from build123d import *


with BuildPart() as part:
    # Sketch1 one side → Revolve1 (revolve)
    with BuildSketch(Plane.XY, mode=Mode.PRIVATE) as revolve1_sk:
        Polygon((0, -3.175), (0, 6.35), (-3.175, 6.35), (-3.175, 5.715), (-2.8575, 5.715), (-2.8575, -2.921), (-2.6035, -3.175), align=None)
    revolve(revolve1_sk.sketch.rotate(Axis((0, 0, 0), (0, 1, 0)), 180), axis=Axis((0, 0, 0), (0, 1, 0)))  # turned: the seam where the file's is

    # Sketch2 → #6-80 Tapped Hole1 (revolve, cut)
    with BuildSketch(Plane(origin=(0, 6.35, 0), x_dir=(0, 0, 1), z_dir=(1, 0, 0))):
        Polygon((0, 0), (0, 9.525), (1.5748, 9.525), (1.3208, 8.911789755), (1.3208, 0.613210245), (1.5748, 0), align=None)
    revolve(axis=Axis((0, 12.7, 0), (0, -1, 0)), mode=Mode.SUBTRACT)


solid = part.part
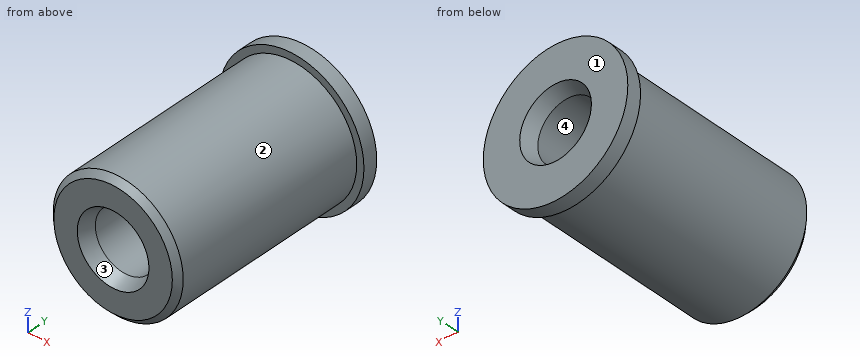
Verification items for the finished model (mm, model axes). Face numbers are marked on the shaded views. Round coordinates to 2 decimals unless told otherwise and drop trailing zeros. Loops run counter-clockwise (first coordinate to the right, second up) from the corner with the lowest first, then second, coordinate; pieces in that order, holes last. Notation, with made-up numbers: (71.25, -8.5) - (84.25, -8.5) arc R21 ccw to (84.25, 23.5) - close; hole circle Ø5 at (-36.75, 10). An arc over 180 degrees is marked (long way). Write item = value, one per line.
Q1. Depth check by flat-ended pin: pin 1 (3 mm diameter, centred on x = -2, y = -2, fed in from -Z); pin 2 (1.5 mm diameter, centred on x = 0.5, y = 2.5, fed in from +Z); pin 3 (2 mm diameter, centred on y = 1.5, z = -0.5, fed in from +X). Enter the tip coordinate at first touch or a pass-through.
Here are the results:
pin_1 = -2.81
pin_2 = 2.86
pin_3 = 2.86
Q2. Mould release check, pull along Z, two halves, no side actions. Record for the marked faces 1, 2, 3 and 4: +Z half, -Z half, draft (parallel to the pull), parting line (faces both ways), or undercut.
Here are the results:
face_1 = draft
face_2 = parting line
face_3 = undercut
face_4 = undercut
Q3. Sectioned sample at C-C on y = 3.5. Record the boundary of the cut face in (x, z) (1 decimal).
Here are the results:
outline = circle Ø5.7 at (0, 0); hole circle Ø2.6 at (0, 0)
Q4. Material ranges on L1, parallel to Z at x = 0, y = -0.75; L2, parallel to Y at x = 2.5, z = 1.75 (3 decimals); L3, parallel to Z at x = -0.5, y = 3.5, recorded low to high.
Here are the results:
L1 = -2.86 to -1.32, 1.32 to 2.86
L2 = 5.715 to 6.35
L3 = -2.81 to -1.22, 1.22 to 2.81
